Can you work these out from the model? Positions are in its coordinate system, mm. Give positions to 0.01 mm unless a question says otherwise; leave off trailing zeros. Order: outer loops, then holes, each group sorted by start corner. A loop starts at its lowest first (then second) coordinate and runs counter-clockwise, first axis right, second up. Notation, with made-up numbers: (-22, -3.75) - (12, -3.75) arc R19 cw to (12, 4.25) - close; hole circle Ø8 at (-5, -0.75). An arc over 180 degrees is marked (long way). Answer as a JSON object with one key per item and string values.
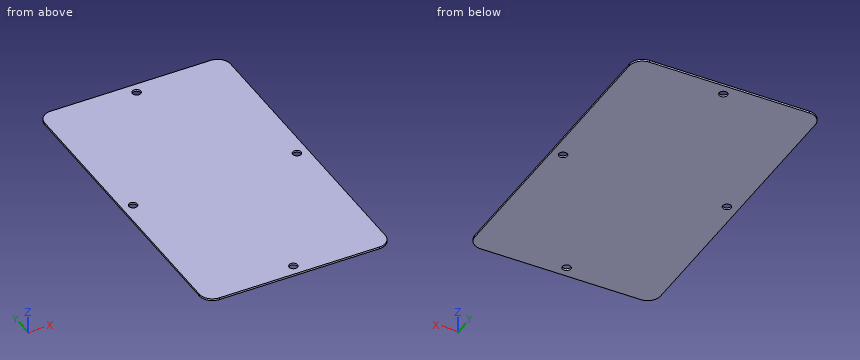
```python
from build123d import *

# Parameters (mm, degrees)
SKETCH1_W          = 144
SKETCH1_H          = 244
BASE_FLANGE1_DEPTH = 1.5
FILLET1_R          = 10
SKETCH6_R          = 3.25
CUT_EXTRUDE1_DEPTH = 10


# Sheet-metal steps are written as plain solids
with BuildPart() as part:
    # Sketch1 → Base-Flange1 (new body)
    with BuildSketch(Plane.XY):
        with Locations((72, 122)):
            Rectangle(SKETCH1_W, SKETCH1_H)
    extrude(amount=-BASE_FLANGE1_DEPTH)

    # Fillet1
    fillet1_edges = [part.edges().sort_by_distance(p)[0] for p in [
        (0, 244, -0.75),
        (144, 244, -0.75),
        (144, 0, -0.75),
        (0, 0, -0.75),
    ]]
    fillet(fillet1_edges, radius=FILLET1_R)

    # Sketch6 → Cut-Extrude1 (cut)
    with BuildSketch(Plane.XY):
        with Locations((72, 235.5)):
            Circle(SKETCH6_R)
        with Locations((72, 8.5)):
            Circle(SKETCH6_R)
        with Locations((8.5, 122)):
            Circle(SKETCH6_R)
        with Locations((135.5, 122)):
            Circle(SKETCH6_R)
    extrude(amount=-CUT_EXTRUDE1_DEPTH, mode=Mode.SUBTRACT)


solid = part.part
```
Q1. I'm going to push a flat-ended pin straight in: pin 1 Ø4 at (x, y) = (135.5, 122) entering from -Z. Where does the tip first touch, or does it pass through?
Recorded:
{"pin 1": "passes through"}
Q2. I need wall thicknesses on L1, parallel to Y at x = 72, z = -0.55; L2, parallel to Y at x = 135.5, z = -0.3. Which ranges of each line are inside material? Lowest first, please.
Recorded:
{"L1": "y = 0 to 5.25, 11.75 to 232.25, 238.75 to 244", "L2": "y = 0.11 to 118.75, 125.25 to 243.89"}
Q3. If we section it at A-A, the plane x = 72: Please give me the cut outline in (y, z), then the cut area to 4 significant figures.
Recorded:
{"outline": "(0, -1.5) - (5.25, -1.5) - (5.25, 0) - (0, 0) - close; (11.75, -1.5) - (232.25, -1.5) - (232.25, 0) - (11.75, 0) - close; (238.75, -1.5) - (244, -1.5) - (244, 0) - (238.75, 0) - close", "area": "346.5 mm^2"}
